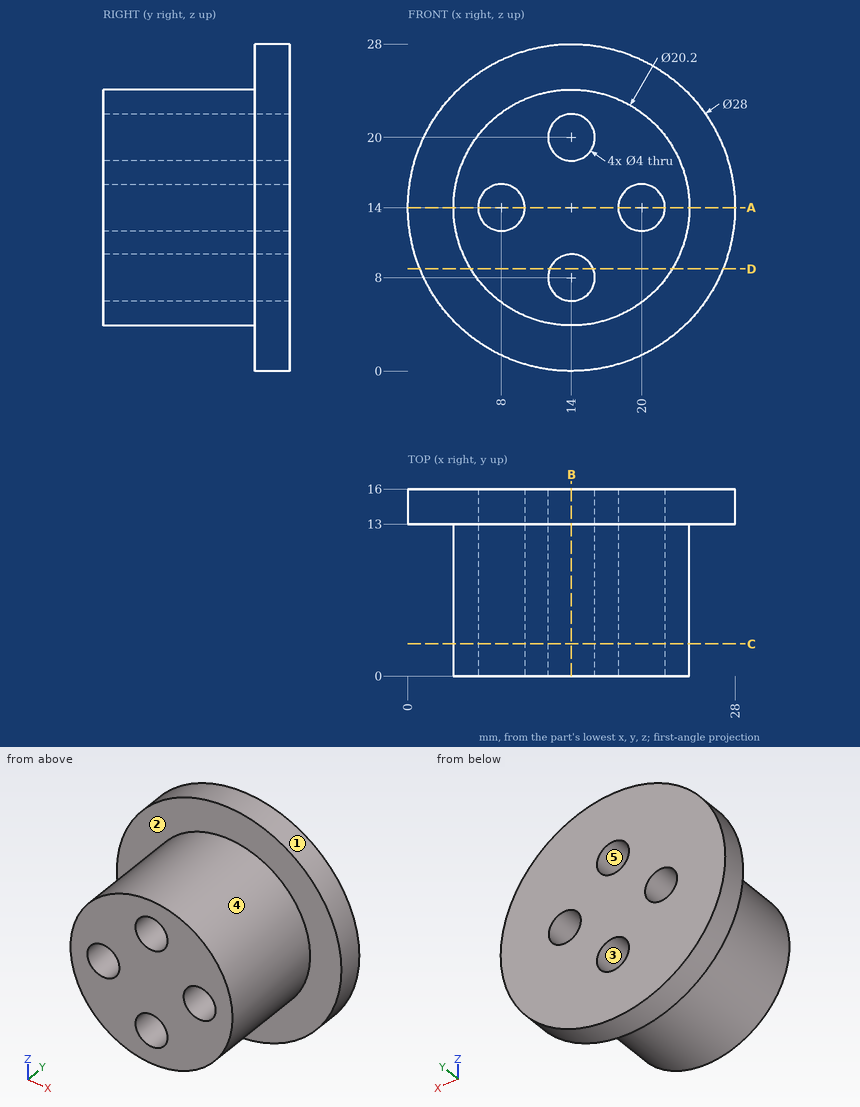
Geometry check sheet. Reference: drawing and pictorial views, mm from the part's lowest x, y, z. A direction names the side the tool comes from. Round coordinates to 2 decimals unless told otherwise and drop trailing zeros. Loops run counter-clockwise (first coordinate to the right, second up) from the corner with the lowest first, then second, coordinate; pieces in that order, holes last. Notation, with made-up numbers: (78.5, 31.25) -> (129.5, 31.25) arc R19 ccw to (129.5, 35.25) -> close; hole circle Ø3 at (40.5, 13). An arc over 180 degrees is marked (long way). Use a Markdown table: item, result.
(1) Scan lines: probe 1 along Z at (x, y) = (14, 9.75); probe 2 along Z at (x, y) = (15.5, 8.5). Record each from-to range of solid material in increasing order.
Calculated:
| item | result |
|---|---|
| probe 1 | 3.9 to 6, 10 to 18, 22 to 24.1 |
| probe 2 | 4.01 to 6.68, 9.32 to 18.68, 21.32 to 23.99 |
(2) Sectioned sample at B-B (x = 14). Enter the section's corners in (y, z).
Calculated:
| item | result |
|---|---|
| outline | (0, 3.9) -> (13, 3.9) -> (13, 0) -> (16, 0) -> (16, 6) -> (0, 6) -> close; (0, 10) -> (16, 10) -> (16, 18) -> (0, 18) -> close; (0, 22) -> (16, 22) -> (16, 28) -> (13, 28) -> (13, 24.1) -> (0, 24.1) -> close |
(3) Sectioned sample at A-A (z = 14). Enter the section's corners in (x, y), then the cut area to 3 significant figures.
Calculated:
| item | result |
|---|---|
| outline | (0, 13) -> (3.9, 13) -> (3.9, 0) -> (6, 0) -> (6, 16) -> (0, 16) -> close; (10, 0) -> (18, 0) -> (18, 16) -> (10, 16) -> close; (22, 0) -> (24.1, 0) -> (24.1, 13) -> (28, 13) -> (28, 16) -> (22, 16) -> close |
| area | 219 mm² |
(4) Sectioned sample at D-D (z = 8.75). Enter the section's corners in (x, y), then the cut area to 3 significant figures.
Calculated:
| item | result |
|---|---|
| outline | (1.02, 13) -> (5.37, 13) -> (5.37, 0) -> (12.15, 0) -> (12.15, 16) -> (1.02, 16) -> close; (15.85, 0) -> (22.63, 0) -> (22.63, 13) -> (26.98, 13) -> (26.98, 16) -> (15.85, 16) -> close |
| area | 243 mm² |
(5) Set-up check for the marked faces 4 and 5: record each of +Z, -Z, +X, -X, +Y, -Y from which the full face is reachable in a straight line by a thin tool's end or side.
Calculated:
| item | result |
|---|---|
| face 4 | -Y |
| face 5 | +Y, -Y |
(6) Go/stop test with flat-tipped pins: P1, Ø3, axis at y = 10, z = 14, coming from the -X side; P2, Ø3, axis at x = 14, z = 8, coming from the +Y side; P3, Ø3, axis at x = 15.5, y = 9.5, coming from the -Z side. Record where each tip stops, or that it passes through.
Calculated:
| item | result |
|---|---|
| P1 | x = 3.9 |
| P2 | through |
| P3 | z = 3.9 |
(7) Mould release check, pull along X, two halves, no side actions. Record for the marked faces 1, 2 and 3: released by +X, released by -X, zero draft, split by the parting line, or undercut.
Calculated:
| item | result |
|---|---|
| face 1 | split by the parting line |
| face 2 | zero draft |
| face 3 | undercut |
(8) Sectioned sample at C-C (y = 2.75). Enter the section's corners in (x, z).
Calculated:
| item | result |
|---|---|
| outline | circle Ø20.2 at (14, 14); hole circle Ø4 at (8, 14); hole circle Ø4 at (14, 8); hole circle Ø4 at (14, 20); hole circle Ø4 at (20, 14) |
